```python
from build123d import *

# Parameters (mm, degrees)
SKETCH1_W           = 60
SKETCH1_H           = 40
BOSS_EXTRUDE1_DEPTH = 3
SKETCH2_W           = 20
SKETCH2_H           = 6
CUT_EXTRUDE1_DEPTH  = 3
SKETCH3_R           = 2
CUT_EXTRUDE2_DEPTH  = 3


with BuildPart() as part:
    # Sketch1 → Boss-Extrude1 (new body)
    with BuildSketch(Plane(origin=(0, 0, 0), x_dir=(1, 0, 0), z_dir=(0, 1, 0))):
        Rectangle(SKETCH1_W, SKETCH1_H)
    extrude(amount=BOSS_EXTRUDE1_DEPTH)

    # Sketch2 → Cut-Extrude1 (cut)
    with BuildSketch(Plane(origin=(0, 3, 0), x_dir=(1, 0, 0), z_dir=(0, 1, 0))):
        with Locations((-20, -20)):
            Rectangle(SKETCH2_W, SKETCH2_H)
        with Locations((20, -20)):
            Rectangle(SKETCH2_W, SKETCH2_H)
        with Locations((20, 20)):
            Rectangle(SKETCH2_W, SKETCH2_H)
        with Locations((-20, 20)):
            Rectangle(SKETCH2_W, SKETCH2_H)
    extrude(amount=-CUT_EXTRUDE1_DEPTH, mode=Mode.SUBTRACT)

    # Sketch3 → Cut-Extrude2 (cut)
    with BuildSketch(Plane(origin=(0, 3, 0), x_dir=(1, 0, 0), z_dir=(0, 1, 0))):
        with Locations(Location((-15, 10, 0), (0, 0, 270))):
            Circle(SKETCH3_R)
        with Locations(Location((-15, -10, 0), (0, 0, 90))):
            Circle(SKETCH3_R)
        with Locations(Location((15, -10, 0), (0, 0, 270))):
            Circle(SKETCH3_R)
        with Locations(Location((15, 10, 0), (0, 0, 90))):
            Circle(SKETCH3_R)
    extrude(amount=-CUT_EXTRUDE2_DEPTH, mode=Mode.SUBTRACT)


solid = part.part
```
Build history of the part. All positions in model axes, mm. A direction names the side the tool comes from. Give positions to 0.01 mm unless a question says otherwise; leave off trailing zeros. Loops run counter-clockwise (first coordinate to the right, second up) from the corner with the lowest first, then second, coordinate; pieces in that order, holes last.
Item 1: Slice it at B-B, the plane y = 1.85. List the corners of the cut face in (x, z).
Answers follow:
outline: (-30, -17) - (-10, -17) - (-10, -20) - (10, -20) - (10, -17) - (30, -17) - (30, 17) - (10, 17) - (10, 20) - (-10, 20) - (-10, 17) - (-30, 17) - close; hole circle Ø4 at (-15, -10); hole circle Ø4 at (-15, 10); hole circle Ø4 at (15, -10); hole circle Ø4 at (15, 10)
Item 2: Which spindle directions (+Z, -Z, +X, -X, +Y, -Y) get a long thin tool onto all of the face, cutting with end or side? Do faces 1 (the face through (10, 2, 19)), 2 (the face through (20, 2, -17)), 3 (the face through (-10, 2, -18)), 4 (the face through (-10, 2, 19)). Say none if no direction does.
Answers follow:
face 1: +Z, +X, +Y, -Y
face 2: -Z, +X, +Y, -Y
face 3: -Z, -X, +Y, -Y
face 4: +Z, -X, +Y, -Y
Item 3: Drill centre lines: line 1 (X direction, y = 0.85, z = -10); line 2 (Z direction, x = -14, y = 2); line 3 (X direction, y = 0.4, z = -17.5). Where is each one in solid material? Low to high.
Answers follow:
line 1: x = -30 to -17, -13 to 13, 17 to 30
line 2: z = -17 to -11.73, -8.27 to 8.27, 11.73 to 17
line 3: x = -10 to 10
Item 4: Slice it at C-C, the plane z = 10. List the corners of the cut face in (x, y), and give its area (3 significant figures).
Answers follow:
outline: (-30, 0) - (-17, 0) - (-17, 3) - (-30, 3) - close; (-13, 0) - (13, 0) - (13, 3) - (-13, 3) - close; (17, 0) - (30, 0) - (30, 3) - (17, 3) - close
area: 156 mm2
Item 5: Slice it at D-D, the plane x = 12. List the corners of the cut face in (y, z), and give its area (3 significant figures).
Answers follow:
outline: (0, -17) - (3, -17) - (3, 17) - (0, 17) - close
area: 102 mm2
Item 6: Pull direction Z, two halves, no side cores. Call faces 5 (the face through (-20, 2, -17)), 6 (the face through (13, 2, -10)), 7 (the face through (20, 2, 17)): released by +Z, released by -Z, zero draft, split by the parting line, or undercut.
Answers follow:
face 5: released by -Z
face 6: undercut
face 7: released by +Z
Item 7: Flat gauge pins, fed straight in: pin 1 (0.9 mm diameter, centred on x = -20, y = 2, fed in from +Z); pin 2 (0.9 mm diameter, centred on y = 2, z = -19, fed in from +X); pin 3 (1.5 mm diameter, centred on x = 20, y = 1, fed in from -Z). Where does each tip first touch, or does it go through?
Answers follow:
pin 1: stops at z = 17
pin 2: stops at x = 10
pin 3: stops at z = -17
Item 8: Slice it at A-A, the plane x = -15. List the corners of the cut face in (y, z).
Answers follow:
outline: (0, -17) - (3, -17) - (3, -12) - (0, -12) - close; (0, -8) - (3, -8) - (3, 8) - (0, 8) - close; (0, 12) - (3, 12) - (3, 17) - (0, 17) - close
